Autodesk Inventor part; units mm, degrees
ref_plane "YZ Plane" through (0, 0, 0) normal (1, 0, 0) x (0, 1, 0)
ref_plane "XZ Plane" through (0, 0, 0) normal (0, 1, 0) x (-1, 0, 0)
ref_plane "XY Plane" through (0, 0, 0) normal (0, 0, 1) x (1, 0, 0)
sketch "Sketch1" plane through (0, 0, 0) normal (0, 1, 0) x (-1, 0, 0)
  circle A0 centre (0, 0) radius 13
  circle A1 centre (0, 0) radius 10.5
  line L0 (0, 13) -> (0, -13)
  point P0 (0, -10.5)
  point P1 (0, 10.5)
  dimension "d0" = 26
  dimension "d1" = 21
extrude "Extrusion1" add sketch "Sketch1" against normal blind 10
extrude "Extrusion2" add sketch "Sketch1" along normal blind 15.5 contours A0 L0 A1 picked at (12.058, 0.9643)
sketch "Sketch2" plane through (0, 15.5, 0) normal (0, 1, 0) x (1, 0, 0)
  circle A0 centre (0, 0) radius 13
  circle A1 centre (0, 0) radius 10.5
  circle A2 centre (0, 0) radius 5
  dimension "d6" = 10
extrude "Extrusion3" add sketch "Sketch2" along normal blind 12 contours A0 | A1
extrude "Extrusion4" cut sketch "Sketch2" along normal blind 15 draft 25 contours A2
sketch "Sketch3" plane through (0, -10, 0) normal (0, -1, 0) x (1, 0, 0)
  line L0 (0, 0) -> (-1.5, 0)
  line L1 (-1.5, 0) -> (-1.5, -12.9132)
  circle A0 centre (0, 0) radius 13
  line L2 (-1.5, 0) -> (-1.5, 12.9132)
  line L3 (0, 0) -> (0, -0.2769)
  line L4 (1.5, 0) -> (1.5, -12.9132)
  line L5 (1.5, 0) -> (1.5, 12.9132)
  point P0 (1.5, -12.9132)
  point P1 (1.5, 12.9132)
  dimension "d11" = 1.5
extrude "Extrusion5" add sketch "Sketch3" along normal blind 38 contours L2 A0 L5 L4 L1
sketch "Sketch6" plane through (0, -10, 0) normal (0, -1, 0) x (1, 0, 0)
  line L0 (-1.5, -12.9132) -> (-1.5, 12.9132)
  arc A0 (-1.5, 12.9132) -> (-1.5, -12.9132) centre (0, 0) ccw
  arc A1 (1.5, -12.9132) -> (1.5, 12.9132) centre (0, 0) ccw
  line L1 (1.5, -12.9132) -> (1.5, 12.9132)
extrude "Extrusion7" add sketch "Sketch6" along normal blind 38 contours A0 L0
sketch "Sketch4" plane through (-1.5, -10, -12.9132) normal (-1, 0, 0) x (0, 0, 1)
  circle A0 centre (12.4097, -33) radius 1.5
  line L0 (25.8263, -38) -> (0, -38)
  circle A1 centre (12.4097, -6) radius 1.5
  point P0 (12.9132, 10)
  dimension "d14" = 5
  dimension "d17" = 3
  dimension "d18" = 3
  dimension "d19" = 27
extrude "Extrusion6" cut sketch "Sketch4" along normal mid plane 30
chamfer "Chamfer1" distance 2 angle 45 1 edges at (1.5, -10, -6.4566)
sketch "Sketch7" plane through (0, -48, 0) normal (0, -1, 0) x (1, 0, 0)
  circle A0 centre (0, 0) radius 13
  line L0 (-10.6184, 7.5) -> (-10.6184, -7.5)
  dimension "d25" = 15
extrude "Extrusion8" cut sketch "Sketch7" against normal blind 38 contours L0 A0 picked at (-11.1206, 1.5629)
properties part number "Tapered guide" material "PC/ABS Plastic"
The listing builds one solid part. Answer for the finished solid, in the listing's coordinates (mm). A direction names the side the tool comes from. Round coordinates to 2 decimals unless told otherwise and drop trailing zeros. Write each loop counter-clockwise with the first axis right and the second up, starting at its lowest first coordinate (ties: lowest second). Pieces come first, ordered by that corner, then holes. Notation, with made-up numbers: (-19, -33.75) - (15, -33.75) arc R18 ccw to (15, -23.75) - close; hole circle Ø10 at (-12, 61.25). An arc over 180 degrees is marked (long way). Use a Markdown table: item, result. Add a question column.
1. The part is cut by section B-B (z = 11.75). Write down the section's boundary in (x, y).
2. A tool of negligible diameter and unlimited length cuts with its end or side. For faces 1 (the face through (7, -10, 0)), 2 (the face through (0, 8, -12)), 3 (the face through (-12, -10, 0)), from which of +Z, -Z, +X, -X, +Y, -Y can it reach the whole face along a straight path? Write none if from no direction.
3. For a pull along Z with two mould halves and no side action, classify faces 4 (the face through (-10.618, -29, 0)), 5 (the face through (-6.7, -28.73, 11.14)), 6 (the face through (-10.5, 7.6, 0.2)) as +Z half, -Z half, draft (parallel to the pull), parting line (faces both ways), or undercut.
4. Flat-ended cylindrical pins translate along their axes: P1, Ø1.2, axis at y = 11, z = -12, coming from the +X side; P2, Ø8, axis at y = 14, z = 8.5, coming from the -X side; P3, Ø8, axis at y = 12.5, z = 2, coming from the -X side; P4, Ø1.2, axis at x = -11.5, z = -2.5, coming from the -Y side. Find the tip coordinate at first contact, or state that the pin passes through.
5. The part is cut by section D-D (y = -40). Write down the section's boundary in (x, z).
6. The part is cut by section A-A (y = -16). Write down the section's boundary in (x, z).
7. Consider line 1 (Z direction, x = -1.5, y = -16); line 2 (Y direction, x = -1, z = -0.5); line 3 (X direction, y = -25, z = -1.5). Determine where each line is inside the solid, lowest interval first.
8. The part is cut by section C-C (y = -8). Write down the section's boundary in (x, z).
Reported:
| question | item | result |
|---|---|---|
| 1 | outline | (-5.56, -48) - (1.5, -48) - (1.5, -12) - (3.5, -10) - (5.56, -10) - (5.56, 0) - (0, 0) - (0, 15.5) - (5.56, 15.5) - (5.56, 27.5) - (-5.56, 27.5) - close |
| 2 | face 1 | +Z, -Z, +X, -Y |
| 2 | face 2 | +Z, -Z, +X |
| 2 | face 3 | +Z, -Z, -X, -Y |
| 3 | face 4 | draft |
| 3 | face 5 | +Z half |
| 3 | face 6 | undercut |
| 4 | P1 | x = 0 |
| 4 | P2 | x = -12.2 |
| 4 | P3 | x = -13 |
| 4 | P4 | y = -10 |
| 5 | outline | (-10.62, -7.5) arc R13 ccw to (1.5, -12.91) - (1.5, 12.91) arc R13 ccw to (-10.62, 7.5) - close |
| 6 | outline | (-10.62, -7.5) arc R13 ccw to (1.5, -12.91) - (1.5, -2) - (-10.62, -2) - close; (-10.62, 1) - (1.5, 1) - (1.5, 12.91) arc R13 ccw to (-10.62, 7.5) - close |
| 7 | line 1 | -12.91 to -2, 1 to 12.91 |
| 7 | line 2 | -48 to -44.5, -41.5 to -17.5, -14.5 to 0 |
| 7 | line 3 | -10.62 to 1.5 |
| 8 | outline | circle Ø26 at (0, 0) |
